Work out the finished part from the listing and answer in its coordinate system (mm). A direction names the side the tool comes from. Give positions to 0.01 mm unless a question says otherwise; leave off trailing zeros. Order: outer loops, then holes, each group sorted by start corner. A loop starts at its lowest first (then second) coordinate and runs counter-clockwise, first axis right, second up.
```python
from build123d import *

# Parameters (mm, degrees)
SKETCH2_W           = 18.40000003
SKETCH2_H           = 2.499999953
SKETCH2_W_2         = 2.000000064
SKETCH2_H_2         = 10.999999971
SKETCH3_R           = 1.75
BOSS_EXTRUDE1_DEPTH = 26


with BuildPart() as part:
    # Sketch2 → Revolve1 (revolve)
    with BuildSketch(Plane.XY):
        with Locations((9.200000015, 1.249999977)):
            Rectangle(SKETCH2_W, SKETCH2_H)
        with Locations((-1.000000032, 5.499999986)):
            Rectangle(SKETCH2_W_2, SKETCH2_H_2)
    revolve(axis=Axis((0, 0, 0), (1, 0, 0)))

    # Sketch3 → Boss-Extrude1 (add)
    with BuildSketch(Plane.ZY.offset(2.000000064)):
        Polygon((0, 23.390158698), (1.5, 23.390158698), (23.390158698, 1.5), (23.390158698, 0), (23.390158698, -1.5), (1.5, -23.390158698), (0, -23.390158698), (-1.5, -23.390158698), (-23.390158698, -1.5), (-23.390158698, 0), (-23.390158698, 1.5), (-1.5, 23.390158698), align=None)
        with Locations((0, 18.384776311)):
            Circle(SKETCH3_R, mode=Mode.SUBTRACT)
        with Locations((18.384776311, 0)):
            Circle(SKETCH3_R, mode=Mode.SUBTRACT)
        with Locations((0, -18.384776311)):
            Circle(SKETCH3_R, mode=Mode.SUBTRACT)
        with Locations((-18.384776311, 0)):
            Circle(SKETCH3_R, mode=Mode.SUBTRACT)
    extrude(amount=BOSS_EXTRUDE1_DEPTH)


solid = part.part
```
1. The part is cut by section C-C (x = -13). Write down the section's boundary in (y, z), then the cut area to 3 significant figures.
Findings below:
outline: (-23.39, -1.5) - (-1.5, -23.39) - (1.5, -23.39) - (23.39, -1.5) - (23.39, 1.5) - (1.5, 23.39) - (-1.5, 23.39) - (-23.39, 1.5) - close; hole circle Ø3.5 at (-18.38, 0); hole circle Ø3.5 at (0, -18.38); hole circle Ø3.5 at (0, 18.38); hole circle Ø3.5 at (18.38, 0)
area: 1,190 mm2
2. The mould has two halves that part along Z. Classify faces 1 (the face through (-28, 0, 0)), 2 (the face through (-14.82, 12.29, -12.6)), 3 (the face through (-14.818, -1.065, -19.774)): pulls with the +Z half, pulls with the -Z half, needs draft (parallel to the pull), parting line crosses it, or undercut.
Findings below:
face 1: needs draft
face 2: pulls with the -Z half
face 3: undercut
3. Which of the six approach directions +Z, -Z, +X, -X, +Y, -Y give full straight-line access (tool end or side, diameter ignored) to faces 4 (the face through (9.329, 2.385, 0.751)), 5 (the face through (-14.82, -12.6, -12.29))?
Findings below:
face 4: +X
face 5: -Z, +X, -X, -Y
4. Given P1, Ø2, axis at x = -22, z = -13, coming from the +Y side; P2, Ø1.5, axis at x = -21, y = -8.5, coming from the -Z side; P3, Ø5, axis at x = -16.5, y = 7, coming from the +Z side, each flat-ended and moving along its own axis, determine where each tip first touches the part or whether it passes through.
Findings below:
P1: stops at y = 12.89
P2: stops at z = -17.14
P3: stops at z = 20.39
5. The part is cut by section D-D (z = 8). Write down the section's boundary in (x, y), then the cut area to 3 significant figures.
Findings below:
outline: (-28, -16.89) - (-2, -16.89) - (-2, -7.55) - (0, -7.55) - (0, 7.55) - (-2, 7.55) - (-2, 16.89) - (-28, 16.89) - close
area: 908 mm2
6. Straight lines are drawn through the part: probe 1 along Y at (x, z) = (-16, 0); probe 2 along Z at (x, y) = (-10, -1); probe 3 along X at (y, z) = (-10.5, -9). For each, find the intervals that lie inside material, in ascending order.
Findings below:
probe 1: y = -23.39 to -20.13, -16.63 to 16.63, 20.13 to 23.39
probe 2: z = -23.39 to -19.82, -16.95 to 16.95, 19.82 to 23.39
probe 3: x = -28 to -2
7. The part is cut by section A-A (y = 0). Write down the section's boundary in (x, z).
Findings below:
outline: (-28, -23.39) - (-2, -23.39) - (-2, -20.13) - (-28, -20.13) - close; (-28, -16.63) - (-2, -16.63) - (-2, -11) - (0, -11) - (0, -2.5) - (18.4, -2.5) - (18.4, 2.5) - (0, 2.5) - (0, 11) - (-2, 11) - (-2, 16.63) - (-28, 16.63) - close; (-28, 20.13) - (-2, 20.13) - (-2, 23.39) - (-28, 23.39) - close
